The listing builds one solid part. Answer for the finished solid, in the listing's coordinates (mm). Coordinates: 2 decimals unless noted, no trailing zeros. Order: outer loops, then holes, each group sorted by start corner. A loop starts at its lowest first (then second) coordinate and runs counter-clockwise, first axis right, second up. Notation, with made-up numbers: (82.25, -19) -> (102.25, -19) arc R6 ccw to (102.25, -9) -> close; hole circle Ø4 at (27, -4.75). An arc over 180 degrees is marked (long way). Write each question's results on one line, items separated by ' | '. Start each with the question number.
(1) Given pin 1 (2 mm diameter, centred on x = 51, z = 2, fed in from +Y); pin 2 (5 mm diameter, centred on x = 26.43, y = -5.5, fed in from +Z); pin 3 (2 mm diameter, centred on x = -3, z = 1.5, fed in from -Y); pin 4 (2 mm diameter, centred on y = -13, z = 1.5, fed in from +X), each flat-ended and moving along its own axis, determine where each tip first touches the part or whether it passes through.
(2) Straight lines are drawn through the part: L1, parallel to X at y = -5.5, z = 2.3; L2, parallel to X at y = -1.25, z = 0.85; L3, parallel to X at y = -10.75, z = 3.1. For each, find the intervals that lie inside material, in ascending order.
(3) The part is cut by section A-A, the plane x = 20.08. Give the vertices of the cut face in (y, z), then the cut area to 3 significant figures.
(4) The part is cut by section D-D, the plane z = 3. Count the separate pieces of the cut face and the enclosed holes in it, then the cut area to 3 significant figures.
(5) The part is cut by section B-B, the plane y = 1.5. Give the vertices of the cut face in (x, z).
(6) The part is cut by section C-C, the plane y = -5.5. Give the vertices of the cut face in (x, z), then the cut area to 3 significant figures.
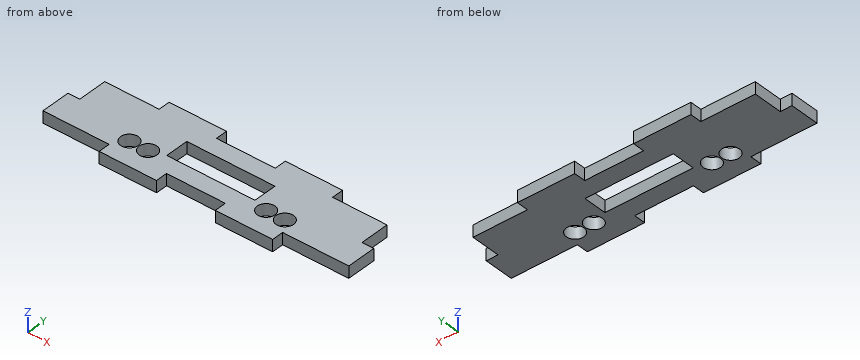
Autodesk Inventor part; units mm, degrees
ref_plane "YZ Plane" through (0, 0, 0) normal (1, 0, 0) x (0, 1, 0)
ref_plane "XZ Plane" through (0, 0, 0) normal (0, 1, 0) x (-1, 0, 0)
ref_plane "XY Plane" through (0, 0, 0) normal (0, 0, 1) x (1, 0, 0)
sketch "Sketch1" plane through (0, 0, 0) normal (0, 0, 1) x (1, 0, 0)
  line L0 (-52, 14) -> (52, 14)
  line L1 (52, 14) -> (52, -14)
  line L2 (52, -14) -> (-52, -14)
  line L3 (-52, -14) -> (-52, 14)
  point P0 (0, 0)
  dimension "d0" = 104
  dimension "d1" = 28
  dimension "d2" = 52
  dimension "d3" = 14
extrude "Base" add sketch "Sketch1" along normal blind 4
sketch "Sketch2" plane through (0, 0, 4) normal (0, 0, 1) x (1, 0, 0)
  line L0 (52, 14) -> (52, -14)
  line L1 (-52, 14) -> (52, 14)
  line L2 (-52, -14) -> (-52, 14)
  line L3 (52, -14) -> (-52, -14)
  line L4 (-52, 14) -> (-29.5, 14)
  line L5 (-29.5, 14) -> (-29.5, 10)
  line L6 (-29.5, 10) -> (-52, 10)
  line L7 (-52, 10) -> (-52, 14)
  line L8 (-52, -10) -> (-29.5, -10)
  line L9 (-29.5, -10) -> (-29.5, -14)
  line L10 (-29.5, -14) -> (-52, -14)
  line L11 (-52, -14) -> (-52, -10)
  line L12 (29.5, -10) -> (52, -10)
  line L13 (52, -10) -> (52, -14)
  line L14 (52, -14) -> (29.5, -14)
  line L15 (29.5, -14) -> (29.5, -10)
  line L16 (29.5, 14) -> (52, 14)
  line L17 (52, 14) -> (52, 10)
  line L18 (52, 10) -> (29.5, 10)
  line L19 (29.5, 10) -> (29.5, 14)
  line L20 (-10, 14) -> (10, 14)
  line L21 (10, 14) -> (10, 10)
  line L22 (10, 10) -> (-10, 10)
  line L23 (-10, 10) -> (-10, 14)
  line L24 (-10, -10) -> (10, -10)
  line L25 (10, -10) -> (10, -14)
  line L26 (10, -14) -> (-10, -14)
  line L27 (-10, -14) -> (-10, -10)
  point P0 (0, 0)
  dimension "d26" = 22.5
  dimension "d27" = 4
  dimension "d28" = 22.5
  dimension "d29" = 4
  dimension "d30" = 22.5
  dimension "d31" = 4
  dimension "d32" = 22.5
  dimension "d33" = 4
  dimension "d34" = 20
  dimension "d35" = 4
  dimension "d36" = 20
  dimension "d37" = 4
  dimension "d38" = 0
  dimension "d39" = 0
  dimension "d40" = 0
  dimension "d41" = 10
  dimension "d42" = 0
  dimension "d43" = 0
  dimension "d44" = 0
  dimension "d45" = 0
  dimension "d46" = 10
  dimension "d47" = 0
  dimension "d48" = 0
  dimension "d49" = 4
extrude "PlatformsPattern" cut sketch "Sketch2" against normal blind 4 contours L0 L18 L19 L1 | L0 L3 L15 L12 | L21 L22 L23 L1 | L5 L6 L2 L1 | L3 L27 L24 L25 | L3 L2 L8 L9
sketch "Sketch3" plane through (0, 0, 4) normal (0, 0, 1) x (1, 0, 0)
  line L0 (52, 10) -> (52, -10)
  line L1 (52, 10) -> (29.5, 10)
  line L2 (-29.5, 10) -> (-52, 10)
  line L3 (-52, -10) -> (-52, 10)
  line L4 (-52, 10) -> (-48, 10)
  line L5 (-48, 10) -> (-48, 0)
  line L6 (-48, 0) -> (-52, 0)
  line L7 (-52, 0) -> (-52, 10)
  line L8 (48, 10) -> (52, 10)
  line L9 (52, 10) -> (52, 0)
  line L10 (52, 0) -> (48, 0)
  line L11 (48, 0) -> (48, 10)
  point P0 (0, 0)
  dimension "d52" = 4
  dimension "d53" = 10
  dimension "d54" = 4
  dimension "d55" = 10
  dimension "d56" = 0
  dimension "d57" = 0
  dimension "d58" = 0
  dimension "d59" = 0
extrude "Sleeves" cut sketch "Sketch3" against normal blind 4
sketch "Sketch4" plane through (0, 0, 4) normal (0, 0, 1) x (1, 0, 0)
  line L0 (-15, 4) -> (15, 4)
  line L1 (15, 4) -> (15, -4)
  line L2 (15, -4) -> (-15, -4)
  line L3 (-15, -4) -> (-15, 4)
  point P0 (0, 0)
  dimension "d62" = 30
  dimension "d63" = 8
  dimension "d66" = 4
  dimension "d72" = 15
extrude "Cabling" cut sketch "Sketch4" against normal blind 4
sketch "Sketch5" plane through (0, 0, 4) normal (0, 0, 1) x (1, 0, 0)
  line L0 (15, 4) -> (15, -4)
  line L1 (52, 0) -> (48, 0)
  line L2 (29.5, -10) -> (52, -10)
  line L3 (52, 0) -> (52, -10)
  line L4 (0, 13.359) -> (0, -17.1065) construction
  point P0 (0, 0)
  point P1 (20.08, -5.5)
  point P2 (26.43, -5.5)
  point P3 (-20.08, -5.5)
  point P4 (-26.43, -5.5)
  dimension "d75" = 5.08
  dimension "d76" = 6.35
  dimension "d78" = 4.5
  dimension "d79" = 5.5
hole "ESCCutout" at (20.08, -5.5, 4) at (26.43, -5.5, 4) at (-20.08, -5.5, 4) at (-26.43, -5.5, 4) direction (0, 0, -1) diameter 6 end through all
properties part number "ShortMiddleStructure"
Established:
1) pin 1: stops at y = 0 | pin 2: passes through | pin 3: stops at y = -10 | pin 4: stops at x = 29.5
2) L1: x = -52 to -29.43, -23.43 to -23.08, -17.08 to 17.08, 23.08 to 23.43, 29.43 to 52 | L2: x = -52 to -15, 15 to 52 | L3: x = -29.5 to -10, 10 to 29.5
3) outline: (-14, 0) -> (-8.5, 0) -> (-8.5, 4) -> (-14, 4) -> close; (-2.5, 0) -> (14, 0) -> (14, 4) -> (-2.5, 4) -> close | area: 88.0 mm^2
4) separate pieces: 1 | enclosed holes: 5 | area: 1,960 mm^2
5) outline: (-48, 0) -> (-15, 0) -> (-15, 4) -> (-48, 4) -> close; (15, 0) -> (48, 0) -> (48, 4) -> (15, 4) -> close
6) outline: (-52, 0) -> (-29.43, 0) -> (-29.43, 4) -> (-52, 4) -> close; (-23.43, 0) -> (-23.08, 0) -> (-23.08, 4) -> (-23.43, 4) -> close; (-17.08, 0) -> (17.08, 0) -> (17.08, 4) -> (-17.08, 4) -> close; (23.08, 0) -> (23.43, 0) -> (23.43, 4) -> (23.08, 4) -> close; (29.43, 0) -> (52, 0) -> (52, 4) -> (29.43, 4) -> close | area: 320 mm^2
